For this review, take the finished solid that the model builds, in its own axes (mm). A direction names the side the tool comes from. Give positions to 0.01 mm unless a question says otherwise; leave off trailing zeros. Use CSV: the item, a comma, the result in double quotes. Start each with the question number.
```python
from build123d import *

# Parameters (mm, degrees)
SKETCH1_W          = 40
SKETCH1_H          = 1.5875
SKETCH2_W          = 25.4
SKETCH2_H          = 12.7
CUT_EXTRUDE1_DEPTH = 155.864521942
CIRPATTERN1_COUNT  = 20


with BuildPart() as part:
    # Sketch1 → Revolve1 (revolve)
    with BuildSketch(Plane.XY, mode=Mode.PRIVATE) as revolve1_sk:
        with Locations((-89.5, 6.57875)):
            Rectangle(SKETCH1_W, SKETCH1_H)
    revolve(revolve1_sk.sketch.rotate(Axis((0, -200069.047495165, 0), (0, 1, 0)), 270), axis=Axis((0, -200069.047495165, 0), (0, 1, 0)))

    # Sketch2 → Cut-Extrude1 (cut, through all)
    with BuildSketch(Plane(origin=(0, 7.3725, 0), x_dir=(1, 0, 0), z_dir=(0, 1, 0))):
        with Locations((0, 93.5)):
            Rectangle(SKETCH2_W, SKETCH2_H)
    cut_extrude1 = extrude(amount=-CUT_EXTRUDE1_DEPTH, mode=Mode.SUBTRACT)

    # CirPattern1: Cut-Extrude1 ×20 about axis
    cirpattern1_axis = Axis((0, 0, 0), (0, 1, 0))
    for i in range(1, CIRPATTERN1_COUNT):
        add(cut_extrude1.rotate(cirpattern1_axis, i * 360 / CIRPATTERN1_COUNT), mode=Mode.SUBTRACT)


solid = part.part
```
1. Clearance check with flat-ended pins moving along their axes: P1, Ø0.5, axis at y = 7, z = -96.5, coming from the +X side; P2, Ø0.8, axis at y = 6.5, z = 93.5, coming from the +X side; P3, Ø0.8, axis at y = 7, z = -93.5, coming from the -X side. State where each tip first meets the part, or that it passes through.
2. Draft analysis for pull direction X (two halves, no side actions). For faces 1 (the face through (-44.631, 6.59, 83.036)), 2 (the face through (-57, 5.785, 41)), 3 (the face through (106.896, 6.59, 23.737)), state which applies: +X half, -X half, draft (parallel to the pull), parting line (faces both ways), or undercut.
3. For faces 4 (the face through (-57, 7.372, 41)), 5 (the face through (83.036, 6.59, -44.631)), list the 3-axis set-ups (+Z, -Z, +X, -X, +Y, -Y) from which the entire face can be reached by the end or side of a thin tool; tool diameter is ignored.
4. To check wall thickness, follow L1, parallel to X at y = 6.35, z = 0; L2, parallel to Z at x = 1.5, y = 6.45. State the ranges of each line that lie inside material, in increasing order. Write a range as [from, to].
5. Consider section A-A (x = 0). State how many separate pieces and enclosed holes the cut face has, plus the area to 3 significant figures.
Answer list:
1,P1,"x = 52.21"
1,P2,"x = 57.64"
1,P3,"x = -57.64"
2,face 1,"undercut"
2,face 2,"draft"
2,face 3,"parting line"
3,face 4,"+Z, -Z, +X, -X, +Y"
3,face 5,"+Y, -Y"
4,L1,"[-109.5, -99.85], [-87.15, -69.5], [69.5, 87.15], [99.85, 109.5]"
4,L2,"[-109.49, -99.85], [-87.15, -69.48], [69.48, 87.15], [99.85, 109.49]"
5,separate pieces,"4"
5,enclosed holes,"0"
5,area,"86.7 mm2"
